Geometry: see drawing. Coordinates: mm, zero at the bounding-box minimum. A direction names the side the tool comes from. Round coordinates to 2 decimals unless told otherwise and drop trailing zeros. Write each loop counter-clockwise with the first axis right and the second up, starting at its lowest first coordinate (ties: lowest second). Pieces come first, ordered by that corner, then holes. Notation, with made-up numbers: (-8.75, 7.25) -> (38.25, 7.25) arc R32 ccw to (38.25, 42.25) -> close; hole circle Ø1 at (-35.75, 51). An arc over 180 degrees is marked (long way). Write item = value, one per line.
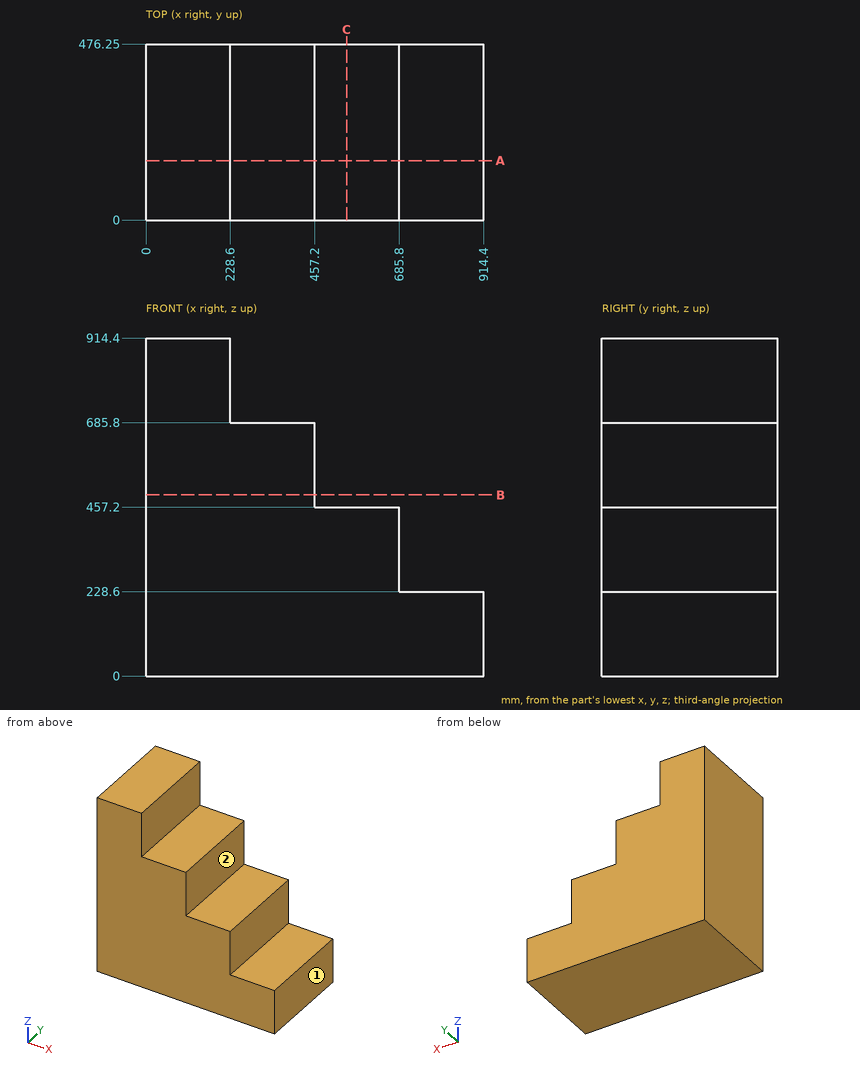
1) Cut plane C-C (x = 543). Return the cut outline in (y, z).
Solutions:
outline = (0, 0) -> (476.25, 0) -> (476.25, 457.2) -> (0, 457.2) -> close
2) Line query: L1, parallel to X at y = 291, z = 354; L2, parallel to Z at x = 749, y = 252.5. Output: solid intervals per line, ascending. Write a range as from..to.
Solutions:
L1 = 0..685.8
L2 = 0..228.6
3) First-contact query: P1, Ø5, axis at x = 357.5, y = 337.5, coming from the +Z side; P2, Ø10, axis at y = 335, z = 501, coming from the +X side; P3, Ø8, axis at x = 771, y = 393.5, coming from the +Z side. Flat tips, straight axial feed; report the tip coordinate or a pass-through.
Solutions:
P1 = 685.8
P2 = 457.2
P3 = 228.6
4) Cut plane B-B (z = 490). Return the cut outline in (x, y).
Solutions:
outline = (0, 0) -> (457.2, 0) -> (457.2, 476.25) -> (0, 476.25) -> close
5) Cut plane A-A (y = 160.5). Return the cut outline in (x, z).
Solutions:
outline = (0, 0) -> (914.4, 0) -> (914.4, 228.6) -> (685.8, 228.6) -> (685.8, 457.2) -> (457.2, 457.2) -> (457.2, 685.8) -> (228.6, 685.8) -> (228.6, 914.4) -> (0, 914.4) -> close
6) Access query for the marked faces 1 and 2. Directions: +Z, -Z, +X, -X, +Y, -Y. A direction counts if a zero-diameter tool reaches every point of the face in a straight line with its end or side. Return the directions, or none.
Solutions:
face_1 = +Z, -Z, +X, +Y, -Y
face_2 = +Z, +X, +Y, -Y
